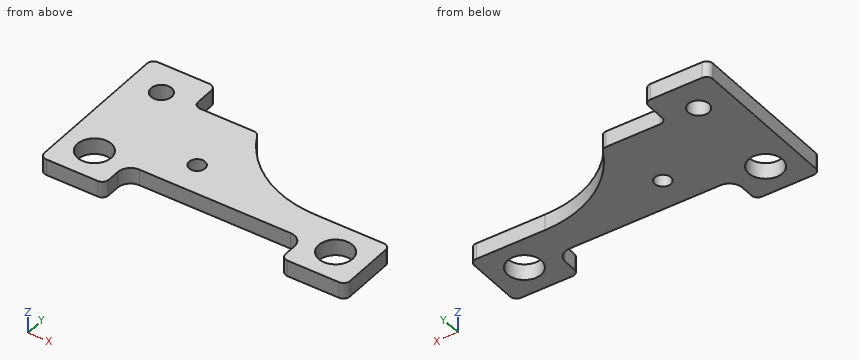
```python
from build123d import *

# Parameters (mm, degrees)
SKETCH1_R           = 5.25
SKETCH1_R_2         = 3.225
SKETCH1_R_3         = 2.5
BOSS_EXTRUDE1_DEPTH = 2.5
FILLET1_R           = 4
FILLET3_R           = 2


with BuildPart() as part:
    # Sketch1 → Boss-Extrude1 (new, symmetric)
    with BuildSketch(Plane.XY):
        with BuildLine():
            Line((-47.5, 0), (-47.5, 50))
            Line((-47.5, 50), (-27.5, 50))
            Line((-27.5, 50), (-27.5, 40))
            Line((-27.5, 40), (-7.5, 40))
            ThreePointArc((-7.5, 40), (5.414502852, 25.418195989), (24.123722991, 19.998004673))
            Line((24.123722991, 19.998004673), (47.5, 19.998004673))
            Line((47.5, 19.998004673), (47.5, -0.001995327))
            Line((47.5, -0.001995327), (27.5, -0.001995327))
            Line((27.5, -0.001995327), (27.5, 10))
            Line((27.5, 10), (-27.5, 10))
            Line((-27.5, 10), (-27.5, 0))
            Line((-27.5, 0), (-47.5, 0))
        make_face()
        with Locations((-37.5, 10)):
            Circle(SKETCH1_R, mode=Mode.SUBTRACT)
        with Locations((-37.5, 40)):
            Circle(SKETCH1_R_2, mode=Mode.SUBTRACT)
        with Locations((-12.5, 20)):
            Circle(SKETCH1_R_3, mode=Mode.SUBTRACT)
        with Locations((37.5, 9.998004673)):
            Circle(SKETCH1_R, mode=Mode.SUBTRACT)
    extrude(amount=BOSS_EXTRUDE1_DEPTH, both=True)

    # Fillet1
    fillet1_edges = [part.edges().sort_by_distance(p)[0] for p in [
        (27.5, 10, 0),
        (-27.5, 10, 0),
    ]]
    fillet(fillet1_edges, radius=FILLET1_R)

    # Fillet3
    fillet3_edges = [part.edges().sort_by_distance(p)[0] for p in [
        (-47.5, 0, 0),
        (-47.5, 50, 0),
        (-27.5, 50, 0),
        (-27.5, 40, 0),
        (-7.5, 40, 0),
        (47.5, 19.998004673, 0),
        (47.5, -0.001995327, 0),
        (27.5, -0.001995327, 0),
        (-27.5, 0, 0),
    ]]
    fillet(fillet3_edges, radius=FILLET3_R)


solid = part.part
```
Build history of the part. All positions in model axes, mm. Round coordinates to 2 decimals unless told otherwise and drop trailing zeros. Write each loop counter-clockwise with the first axis right and the second up, starting at its lowest first coordinate (ties: lowest second). Pieces come first, ordered by that corner, then holes. Notation, with made-up numbers: (-13.5, -22) -> (31.5, -22) arc R23 ccw to (31.5, -1) -> close; hole circle Ø4 at (56.25, 84.5). An arc over 180 degrees is marked (long way). Put each result on its own line as item: value.
Item 1: Slice it at C-C, the plane z = -0.15. Give the cut face in (x, y) (3 decimals), plus the area to 3 significant figures.
Here are the results:
outline: (-47.5, 2) arc R2 ccw to (-45.5, 0) -> (-29.5, 0) arc R2 ccw to (-27.5, 2) -> (-27.5, 6) arc R4 cw to (-23.5, 10) -> (23.5, 10) arc R4 cw to (27.5, 6) -> (27.5, 1.998) arc R2 ccw to (29.5, -0.002) -> (45.5, -0.002) arc R2 ccw to (47.5, 1.998) -> (47.5, 17.998) arc R2 ccw to (45.5, 19.998) -> (24.124, 19.998) arc R35 cw to (-6.964, 38.919) arc R2 ccw to (-8.741, 40) -> (-25.5, 40) arc R2 cw to (-27.5, 42) -> (-27.5, 48) arc R2 ccw to (-29.5, 50) -> (-45.5, 50) arc R2 ccw to (-47.5, 48) -> close; hole circle Ø10.5 at (-37.5, 10); hole circle Ø6.45 at (-37.5, 40); hole circle Ø5 at (-12.5, 20); hole circle Ø10.5 at (37.5, 9.998)
area: 2,300 mm^2
Item 2: Slice it at D-D, the plane x = 37.5. Give the cut face in (y, z), plus the area to 3 significant figures.
Here are the results:
outline: (0, -2.5) -> (4.75, -2.5) -> (4.75, 2.5) -> (0, 2.5) -> close; (15.25, -2.5) -> (20, -2.5) -> (20, 2.5) -> (15.25, 2.5) -> close
area: 47.5 mm^2
Item 3: Slice it at B-B, the plane x = -12.5. Give the cut face in (y, z), plus the area to 3 significant figures.
Here are the results:
outline: (10, -2.5) -> (17.5, -2.5) -> (17.5, 2.5) -> (10, 2.5) -> close; (22.5, -2.5) -> (40, -2.5) -> (40, 2.5) -> (22.5, 2.5) -> close
area: 125 mm^2
Item 4: Flat gauge pins, fed straight in: P1, Ø8.5, axis at x = 37.5, y = 10, coming from the +Z side; P2, Ø1.5, axis at x = 6, z = 0.5, coming from the -Y side; P3, Ø1.5, axis at x = 34, z = -1, coming from the +Y side. Where does each tip first touch, or does it go through?
Here are the results:
P1: passes through
P2: stops at y = 10
P3: stops at y = 20
Item 5: Wall check: probe 1 along Y at (x, z) = (-37.5, -1.2) (3 decimals); probe 2 along X at (y, z) = (9.5, -1.3); probe 3 along X at (y, z) = (6.5, 2.25). Give the ranges that are in metal, low to high. Write a range as from..to.
Here are the results:
probe 1: y = 0..4.75, 15.25..36.775, 43.225..50
probe 2: x = -47.5..-42.73, -32.27..-25.44, 25.44..32.27, 42.73..47.5
probe 3: x = -47.5..-41.41, -33.59..-27.47, 27.47..33.59, 41.41..47.5
Item 6: Slice it at A-A, the plane x = -37.5. Give the cut face in (y, z) (3 decimals).
Here are the results:
outline: (0, -2.5) -> (4.75, -2.5) -> (4.75, 2.5) -> (0, 2.5) -> close; (15.25, -2.5) -> (36.775, -2.5) -> (36.775, 2.5) -> (15.25, 2.5) -> close; (43.225, -2.5) -> (50, -2.5) -> (50, 2.5) -> (43.225, 2.5) -> close
